```python
from build123d import *

# Parameters (mm, degrees)
SKETCH2_W               = 5
SKETCH2_H               = 33.382597824
CUT_EXTRUDE1_DEPTH      = 11
CUT_EXTRUDE1_DEPTH_BACK = 11
SKETCH3_R               = 5
CUT_EXTRUDE2_DEPTH      = 13.5
CUT_EXTRUDE2_DEPTH_BACK = 8.5


with BuildPart() as part:
    # Sketch1 → Revolve1 (revolve)
    with BuildSketch(Plane(origin=(0, 0, 2.5), x_dir=(-1, 0, 0), z_dir=(0, 0, -1))):
        with BuildLine():
            Line((0, 233.5), (0, 83.5))
            ThreePointArc((0, 83.5), (7.071067812, 86.428932188), (10, 93.5))
            Line((10, 93.5), (10, 233.5))
            Line((10, 233.5), (0, 233.5))
        make_face()
    revolve(axis=Axis((0, 233.5, 2.5), (0, -1, 0)))

    # Sketch2 → Cut-Extrude1 (cut, two sides)
    with BuildSketch(Plane(origin=(0, 0, 0), x_dir=(0, 0, -1), z_dir=(1, 0, 0))) as cut_extrude1_sk:
        with Locations((-2.5, 91.70929716)):
            Rectangle(SKETCH2_W, SKETCH2_H)
    extrude(amount=CUT_EXTRUDE1_DEPTH, mode=Mode.SUBTRACT)
    extrude(cut_extrude1_sk.sketch, amount=-CUT_EXTRUDE1_DEPTH_BACK, mode=Mode.SUBTRACT)

    # Sketch3 → Cut-Extrude2 (cut, two sides)
    with BuildSketch(Plane.XY) as cut_extrude2_sk:
        with Locations((0, 92.5)):
            Circle(SKETCH3_R)
    extrude(amount=CUT_EXTRUDE2_DEPTH, mode=Mode.SUBTRACT)
    extrude(cut_extrude2_sk.sketch, amount=-CUT_EXTRUDE2_DEPTH_BACK, mode=Mode.SUBTRACT)


solid = part.part
```
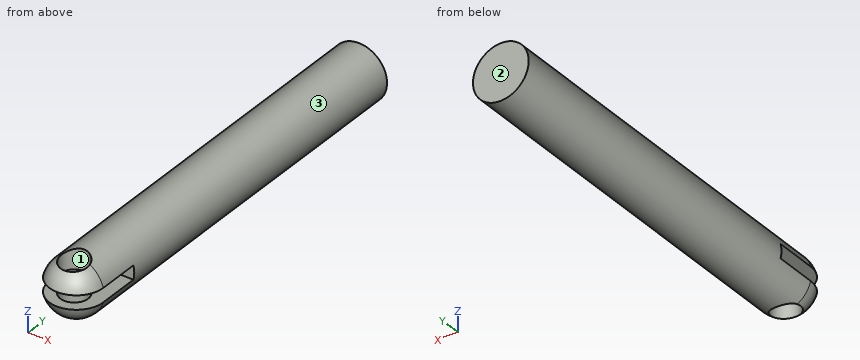
Can you work these out from the model? Positions are in its coordinate system, mm. Face numbers are marked on the shaded views. Round coordinates to 2 decimals unless told otherwise and drop trailing zeros. Order: outer loops, then holes, each group sorted by start corner. A loop starts at its lowest first (then second) coordinate and runs counter-clockwise, first axis right, second up.
(1) If we section it at A-A (x = 0): Please give me the cut outline in (y, z), plus the area to 3 significant figures.
Results are:
outline: (83.82, 0) arc R10 ccw to (87.5, -5.5) - (87.5, 0) - close; (83.82, 5) - (87.5, 5) - (87.5, 10.5) arc R10 ccw to start; (97.5, -7.5) - (233.5, -7.5) - (233.5, 12.5) - (97.5, 12.5) - (97.5, 5) - (108.4, 5) - (108.4, 0) - (97.5, 0) - close
area: 2,690 mm2
(2) I'm going to push flat-ended pins straight in: pin 1 (8 mm diameter, centred on y = 127.5, z = 7, fed in from -X); pin 2 (4 mm diameter, centred on y = 199, z = -2, fed in from -X); pin 3 (1 mm diameter, centred on y = 135.5, z = 10, fed in from +X). Where does each tip first touch, or does it pass through?
Results are:
pin 1: stops at x = -9.99
pin 2: stops at x = -9.68
pin 3: stops at x = 7.14
(3) We'd pull the mould along X, two halves only. Please class the marked faces 1, 2 and 3: +X half, -X half, draft (parallel to the pull), parting line (faces both ways), or undercut.
Results are:
face 1: undercut
face 2: draft
face 3: parting line
(4) If we section it at D-D (y = 165.5): Please give me the cut outline in (x, z), plus the area to 3 significant figures.
Results are:
outline: circle Ø20 at (0, 2.5)
area: 314 mm2
(5) If we section it at B-B (z = 6.25): Please give me the cut outline in (x, y).
Results are:
outline: (-9.27, 93.5) arc R9.27 ccw to (9.27, 93.5) - (9.27, 233.5) - (-9.27, 233.5) - close; hole circle Ø10 at (0, 92.5)
(6) If I drill on L1, parallel to Y at x = 2, z = 7; L2, parallel to Y at x = -2.25, z = 9; L3, parallel to X at y = 160, z = 0, over which ranges is the centre line in solid material (lowest first)?
Results are:
L1: y = 84.8 to 87.92, 97.08 to 233.5
L2: y = 86.24 to 88.03, 96.97 to 233.5
L3: x = -9.68 to 9.68
(7) If we section it at C-C (x = 6.5): Please give me the cut outline in (y, z).
Results are:
outline: (86.32, 0) arc R7.6 ccw to (93.5, -5.1) - (233.5, -5.1) - (233.5, 10.1) - (93.5, 10.1) arc R7.6 ccw to (86.32, 5) - (108.4, 5) - (108.4, 0) - close
